Check sheet for the modelled part. Datum: model origin and axes. Units: mm. A direction names the side the tool comes from. Give positions to 0.01 mm unless a question says otherwise; leave off trailing zeros. Write each loop counter-clockwise with the first axis right and the second up, starting at its lowest first coordinate (ties: lowest second). Pieces come first, ordered by that corner, then holes.
Autodesk Inventor part; units mm, degrees
ref_plane "Work Plane3" through (0, 19.685, 0) normal (0, 1, 0) x (-1, 0, 0)
ref_plane "Work Plane5" through (0, 0, 0) normal (0, 0, 1) x (1, 0, 0)
ref_plane "YZ Plane" through (0, 0, 0) normal (1, 0, 0) x (0, 1, 0)
sketch "Sketch1" plane through (0, 0, 0) normal (0, 0, 1) x (1, 0, 0)
  circle A0 centre (-21.4074, 14.2963) radius 6.35
  circle A1 centre (-21.4074, 14.2963) radius 3.175
  point P0 (0, 0)
  dimension "d0" = 12.7
  dimension "d1" = 6.35
extrude "Extrusion1" add sketch "Sketch1" along normal blind 12.7
sketch "Sketch2" plane through (-21.4074, 14.2963, 0) normal (0, 0, -1) x (-1, 0, 0)
  circle A0 centre (0, 0) radius 3.175
  circle A1 centre (0, 0) radius 6.35
  circle A2 centre (0, 0) radius 5.3975
  point P0 (-21.4074, -14.2963)
  dimension "d4" = 10.795
extrude "Extrusion2" add sketch "Sketch2" along normal blind 25.4 contours A2
sketch "Sketch3" plane through (-21.4074, 14.2963, -25.4) normal (0, 0, -1) x (-1, 0, 0)
  circle A0 centre (0, 0) radius 3.175
  circle A1 centre (0, 0) radius 5.3975
  circle A2 centre (0, 0) radius 6.35
  point P0 (-21.4074, -14.2963)
  dimension "d7" = 12.7
extrude "Extrusion3" add sketch "Sketch3" along normal blind 12.7 contours A1 | A2
ref_plane "Work Plane3" through (0, 19.685, 0) normal (0, 1, 0) x (-1, 0, 0)
sketch "Sketch4" plane through (0, 19.685, 0) normal (0, 1, 0) x (-1, 0, 0)
  line L0 (26.8049, -25.4) -> (16.0099, -25.4)
  line L1 (26.8049, 0) -> (16.0099, 0)
  line L2 (26.8049, 0) -> (26.8049, -25.4)
  line L3 (16.0099, 0) -> (16.0099, -25.4)
  circle A0 centre (21.4074, -12.7) radius 5.3975
  circle A1 centre (21.4074, -12.7) radius 3.175
  point P0 (0, 0)
  dimension "d13" = 6.35
extrude "Extrusion4" add sketch "Sketch4" against normal blind 23.495 contours A0
sketch "Sketch5" plane through (-21.4074, -3.81, -12.7) normal (0, -1, 0) x (1, 0, 0)
  circle A0 centre (0, 0) radius 3.175
  circle A1 centre (0, 0) radius 5.3975
  circle A2 centre (0, 0) radius 6.35
  point P0 (21.4074, 12.7)
  dimension "d16" = 12.7
extrude "Extrusion5" add sketch "Sketch5" along normal blind 12.7 contours A1 | A2
ref_plane "Work Plane5" through (0, 0, 0) normal (0, 0, 1) x (1, 0, 0)
sketch "Sketch7" plane through (0, 0, 0) normal (0, 0, 1) x (1, 0, 0)
  circle A0 centre (-21.4074, 14.2963) radius 5.3975
  circle A1 centre (-21.4074, 14.2963) radius 5.3975
  line L0 (-16.0099, 19.6938) -> (-26.8049, 19.6938)
  line L1 (-26.8049, 19.6938) -> (-26.8049, 8.8988)
  line L2 (-26.8049, 8.8988) -> (-16.0099, 8.8988)
  line L3 (-16.0099, 8.8988) -> (-16.0099, 19.6938)
  line L4 (-16.0099, 14.2963) -> (-26.8049, 14.2963)
  line L5 (-16.0099, 14.2963) -> (-26.8049, 14.2963)
  line L6 (-26.8049, 14.2963) -> (-26.8049, 8.8988)
  line L7 (-26.8049, 8.8988) -> (-16.0099, 8.8988)
  line L8 (-16.0099, 8.8988) -> (-16.0099, 14.2963)
  arc A2 (-26.8049, 14.2963) -> (-16.0099, 14.2963) centre (-21.4074, 14.2963) ccw
  line L9 (-16.0099, 19.6938) -> (-26.8049, 19.6938)
  line L10 (-26.8049, 19.6938) -> (-26.8049, 14.2963)
  line L11 (-26.8049, 14.2963) -> (-16.0099, 14.2963)
  line L12 (-16.0099, 14.2963) -> (-16.0099, 19.6938)
  arc A3 (-16.0099, 14.2963) -> (-26.8049, 14.2963) centre (-21.4074, 14.2963) ccw
  point P0 (0, 0)
extrude "Extrusion7" cut sketch "Sketch7" against normal blind 25.4 contours A0 L0 L3 | A0 L1 L0
properties part number "Joiner Base 1764"
1) Access from +Z, -Z, +X, -X, +Y, -Y to the whole of each face (thin tool, end or side, straight path). Record for faces 1 (the cylindrical face through (-24.34, 15.51, -27.43)), 2 (the flat face through (-19, 9, -25.4)), 3 (the cylindrical face through (-15.35, 12.39, 6.26)).
2) Sectioned sample at A-A on z = -26.5. Record the boundary of the cut face in (x, y) (3 decimals), then the cut area to 3 significant figures.
3) Draft check along Y on faces 4 (the cylindrical face through (-20.58, 8, -31.66)), 5 (the cylindrical face through (-21.338, 14.341, -15.874)), 6 (the flat face through (-26, 18, 0)). Enter one of: +Y half, -Y half, draft (parallel to the pull), parting line (faces both ways), or undercut.
4) Sectioned sample at C-C on x = -17.25. Record the boundary of the cut face in (y, z), then the cut area to 3 significant figures.
5) Scan lines: L1, parallel to X at y = 14.5, z = -30; L2, parallel to Y at x = -19.25, z = -7.5; L3, parallel to Z at x = -22.75, y = -14.5. Record each from-to range of solid material in increasing order.
6) Sectioned sample at D-D on y = -11.5. Record the boundary of the cut face in (x, z) (3 decimals), then the cut area to 3 significant figures.
7) Gauge pin test, flat ends, axial feed: pin 1 (3 mm diameter, centred on y = 6.5, z = -10.5, fed in from -X); pin 2 (2 mm diameter, centred on x = -20, z = -32.5, fed in from -Y); pin 3 (3 mm diameter, centred on x = -22, z = -12.5, fed in from +Y); pin 4 (7.5 mm diameter, centred on x = -21.41, y = 14.3, fed in from -Z). Record the tip position at first contact, or that the pin passes through.
Answers below:
1. face 1: -Z
1. face 2: none
1. face 3: +Z
2. outline: circle Ø12.7 at (-21.407, 14.296); hole circle Ø6.35 at (-21.407, 14.296)
2. area: 95.0 mm2
3. face 4: parting line
3. face 5: undercut
3. face 6: draft
4. outline: (-16.51, -17.5) - (-3.81, -17.5) - (-3.81, -16.14) - (10.85, -16.14) - (10.85, -25.4) - (9.5, -25.4) - (9.5, -38.1) - (19.1, -38.1) - (19.1, -25.4) - (17.74, -25.4) - (17.74, 0) - (19.1, 0) - (19.1, 12.7) - (9.5, 12.7) - (9.5, 0) - (10.85, 0) - (10.85, -9.26) - (-3.81, -9.26) - (-3.81, -7.9) - (-16.51, -7.9) - close
4. area: 642 mm2
5. L1: x = -27.75 to -24.58, -18.24 to -15.06
5. L2: y = -16.51 to -3.81, 9.35 to 11.97, 16.63 to 19.24
5. L3: z = -18.91 to -15.58, -9.82 to -6.49
6. outline: circle Ø12.7 at (-21.407, -12.7); hole circle Ø6.35 at (-21.407, -12.7)
6. area: 95.0 mm2
7. pin 1: stops at x = -26.76
7. pin 2: stops at y = 7.96
7. pin 3: stops at y = 19.69
7. pin 4: stops at z = -38.1
